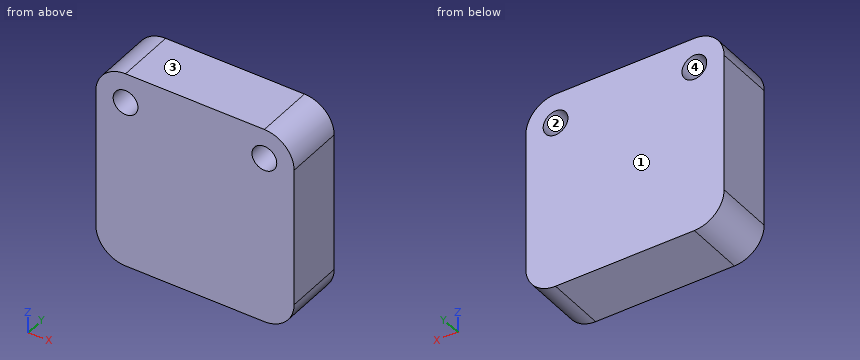
```python
from build123d import *

# Parameters (mm, degrees)
SKETCH1_W               = 20
SKETCH1_H               = 20
BOSS_EXTRUDE1_DEPTH     = 6
FILLET1_R               = 3
SKETCH2_R               = 1.25
CUT_EXTRUDE1_DEPTH      = 1
CUT_EXTRUDE1_DEPTH_BACK = 7


with BuildPart() as part:
    # Sketch1 → Boss-Extrude1 (new body)
    with BuildSketch(Plane(origin=(0, 0, 0), x_dir=(1, 0, 0), z_dir=(0, 1, 0))):
        with Locations((10, 10)):
            Rectangle(SKETCH1_W, SKETCH1_H)
    extrude(amount=BOSS_EXTRUDE1_DEPTH)

    # Fillet1
    fillet1_edges = [part.edges().sort_by_distance(p)[0] for p in [
        (0, 3, -20),
        (20, 3, -20),
        (20, 3, 0),
        (0, 3, 0),
    ]]
    fillet(fillet1_edges, radius=FILLET1_R)

    # Sketch2 → Cut-Extrude1 (cut, two sides)
    with BuildSketch(Plane(origin=(0, 6, 0), x_dir=(1, 0, 0), z_dir=(0, 1, 0))) as cut_extrude1_sk:
        with Locations((3, 3)):
            Circle(SKETCH2_R)
        with Locations((17, 3)):
            Circle(SKETCH2_R)
    extrude(amount=CUT_EXTRUDE1_DEPTH, mode=Mode.SUBTRACT)
    extrude(cut_extrude1_sk.sketch, amount=-CUT_EXTRUDE1_DEPTH_BACK, mode=Mode.SUBTRACT)


solid = part.part
```
Verification items for the finished model (mm, model axes). Face numbers are marked on the shaded views. Round coordinates to 2 decimals unless told otherwise and drop trailing zeros. Loops run counter-clockwise (first coordinate to the right, second up) from the corner with the lowest first, then second, coordinate; pieces in that order, holes last. Notation, with made-up numbers: (53, 3.5) -> (97, 3.5) arc R26 cw to (97, 38.5) -> close; hole circle Ø10 at (32.5, -10.75). An arc over 180 degrees is marked (long way). Answer as a JSON object with one key per item and string values.
Q1. Section check A-A (y = 4.1). Record the boundary of the cut face in (x, z), then the cut area to 3 significant figures.
Data:
{"outline": "(0, -17) arc R3 ccw to (3, -20) -> (17, -20) arc R3 ccw to (20, -17) -> (20, -3) arc R3 ccw to (17, 0) -> (3, 0) arc R3 ccw to (0, -3) -> close; hole circle Ø2.5 at (3, -3); hole circle Ø2.5 at (17, -3)", "area": "382 mm2"}
Q2. Section check C-C (x = 1.5). Record the boundary of the cut face in (y, z), then the cut area to 3 significant figures.
Data:
{"outline": "(0, -19.6) -> (6, -19.6) -> (6, -0.4) -> (0, -0.4) -> close", "area": "115 mm2"}
Q3. Go/stop test with a flat-tipped pin: P1, Ø2, axis at x = 17, z = -3, coming from the -Y side. Record where the tip stops, or that it passes through.
Data:
{"P1": "passes through"}
Q4. Scan lines: line 1 (Z direction, x = 17, y = 2.95); line 2 (X direction, y = 2.7, z = -3.5); line 3 (Z direction, x = 18.75, y = 4.45). Record each from-to range of solid material in increasing order. Write a range as from..to.
Data:
{"line 1": "z = -20..-4.25, -1.75..0", "line 2": "x = 0..1.85, 4.15..15.85, 18.15..20", "line 3": "z = -19.44..-0.56"}
Q5. Section check B-B (x = 16.5). Record the boundary of the cut face in (y, z), then the cut area to 3 significant figures.
Data:
{"outline": "(0, -20) -> (6, -20) -> (6, -4.15) -> (0, -4.15) -> close; (0, -1.85) -> (6, -1.85) -> (6, 0) -> (0, 0) -> close", "area": "106 mm2"}
Q6. Draft check along Z on the marked faces 1, 2, 3 and 4. Enter one of: pulls with the +Z half, pulls with the -Z half, needs draft (parallel to the pull), parting line crosses it, or undercut.
Data:
{"face 1": "needs draft", "face 2": "undercut", "face 3": "pulls with the +Z half", "face 4": "undercut"}
